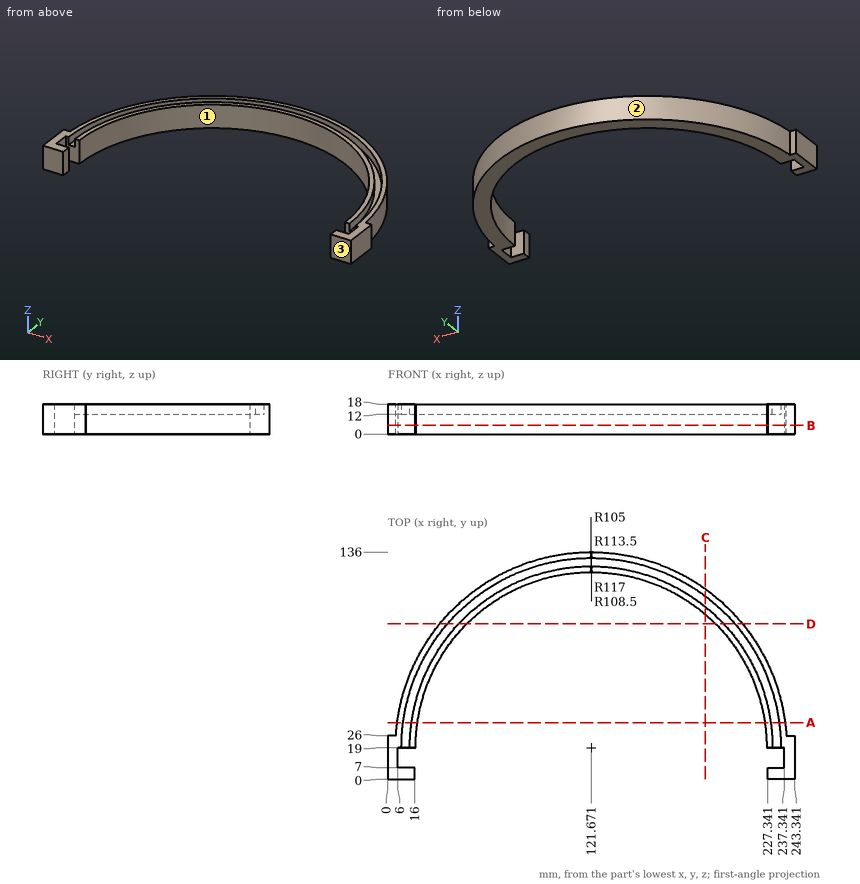
Study the drawing (mm; zero at the part's minimum x, y, z) and answer. Round coordinates to 2 decimals unless told otherwise and drop trailing zeros. Write each loop counter-clockwise with the first axis right and the second up, starting at its lowest first coordinate (ties: lowest second). Pieces come first, ordered by that corner, then holes.
1) The mould has two halves that part along X. Classify the marked faces 1, 2 and 3: pulls with the +X half, pulls with the -X half, needs draft (parallel to the pull), parting line crosses it, or undercut.
2) A cutting plane is placed at B-B (z = 5.25). Give the vertices of the cut face in (x, y).
3) Given pin 1 Ø4 at (x, z) = (77.5, 3) entering from +Y (1 decimal); pin 2 Ø5.5 at (x, z) = (2, 6) entering from +Y; pin 3 Ø10 at (x, z) = (192, 11.5) entering from +Y, each flat-ended and moving along its own axis, determine where each tip first touches the part or whether it passes through.
4) A cutting plane is placed at C-C (x = 190). Give the vertices of the cut face in (y, z) (1 decimal), plus the area to 3 significant figures.
5) Straight lines are drawn through the part: line 1 (X direction, y = 66.5, z = 16.75) (1 decimal); line 2 (X direction, y = 27.5, z = 14.5) (1 decimal); line 3 (X direction, y = 13, z = 8). For each, find the intervals that lie inside material, in ascending order.
6) A cutting plane is placed at A-A (y = 34). Give the vertices of the cut face in (x, z) (1 decimal).
7) A cutting plane is placed at D-D (y = 93). Give the vertices of the cut face in (x, z) (1 decimal), plus the area to 3 significant figures.
Completed:
1. face 1: undercut
1. face 2: parting line crosses it
1. face 3: needs draft
2. outline: (0, 0) - (16, 0) - (16, 7) - (6, 7) - (6, 19) - (16.67, 19) arc R105 cw to (226.67, 19) - (237.34, 19) - (237.34, 7) - (227.34, 7) - (227.34, 0) - (243.34, 0) - (243.34, 26) - (238.46, 26) arc R117 ccw to (4.88, 26) - (0, 26) - close
3. pin 1: stops at y = 128.1
3. pin 2: stops at y = 26
3. pin 3: stops at y = 116.06
4. outline: (98.7, 0) - (114, 0) - (114, 18) - (109.6, 18) - (109.6, 12) - (103.3, 12) - (103.3, 18) - (98.7, 18) - close
4. area: 236 mm2
5. line 1: x = 14.7 to 18.6, 24.1 to 28, 215.3 to 219.2, 224.8 to 228.6
5. line 2: x = 5 to 8.5, 13.5 to 17, 226.3 to 229.8, 234.9 to 238.4
5. line 3: x = 0 to 6, 237.34 to 243.34
6. outline: (5.6, 0) - (17.7, 0) - (17.7, 18) - (14.2, 18) - (14.2, 12) - (9.2, 12) - (9.2, 18) - (5.6, 18) - close; (225.6, 0) - (237.7, 0) - (237.7, 18) - (234.2, 18) - (234.2, 12) - (229.1, 12) - (229.1, 18) - (225.6, 18) - close
7. outline: (31, 0) - (47.2, 0) - (47.2, 18) - (42.3, 18) - (42.3, 12) - (35.6, 12) - (35.6, 18) - (31, 18) - close; (196.2, 0) - (212.3, 0) - (212.3, 18) - (207.7, 18) - (207.7, 12) - (201, 12) - (201, 18) - (196.2, 18) - close
7. area: 500 mm2
